Verification items for the finished model (mm, model axes). Face numbers are marked on the shaded views. A direction names the side the tool comes from. Coordinates: 2 decimals unless noted, no trailing zeros. Order: outer loops, then holes, each group sorted by start corner. A loop starts at its lowest first (then second) coordinate and runs counter-clockwise, first axis right, second up. Notation, with made-up numbers: (67.25, -1.5) -> (117.25, -1.5) arc R21 ccw to (117.25, 33.5) -> close; hole circle Ø10 at (-8.5, -32). An arc over 180 degrees is marked (long way). Write item = value, one per line. Start each with the question number.
from build123d import *

# Parameters (mm, degrees)
SKETCH1_W           = 8.89
SKETCH1_H           = 11.2776
SKETCH1_R           = 2.54
BOSS_EXTRUDE1_DEPTH = 2.54
SKETCH4_W           = 17.78
SKETCH4_H           = 11.43
SKETCH4_R           = 2.54
BOSS_EXTRUDE2_DEPTH = 2.54


with BuildPart() as part:
    # Sketch1 → Boss-Extrude1 (new body)
    with BuildSketch(Plane(origin=(0, 0, 0), x_dir=(1, 0, 0), z_dir=(0, 1, 0))):
        with Locations((-4.445, -5.6388)):
            Rectangle(SKETCH1_W, SKETCH1_H)
        with Locations((-4.445, -4.3688)):
            Circle(SKETCH1_R, mode=Mode.SUBTRACT)
    extrude(amount=BOSS_EXTRUDE1_DEPTH)

    # Sketch4 → Boss-Extrude2 (add)
    with BuildSketch(Plane.XY.offset(11.2776)):
        with Locations((-8.89, 5.715)):
            Rectangle(SKETCH4_W, SKETCH4_H)
        with Locations((-13.335, 6.985)):
            Circle(SKETCH4_R, mode=Mode.SUBTRACT)
    extrude(amount=-BOSS_EXTRUDE2_DEPTH)


solid = part.part
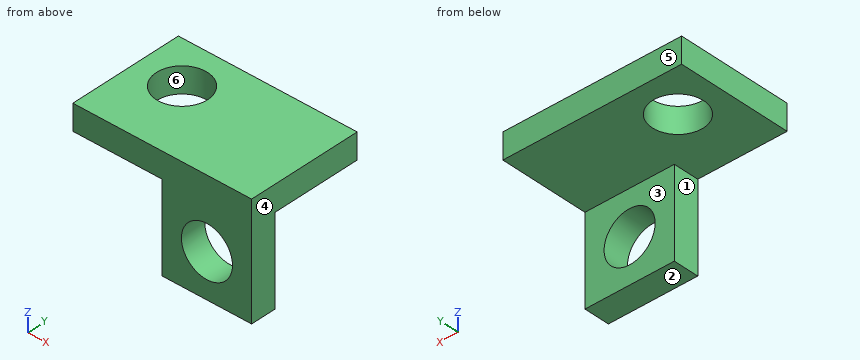
Item 1: Section check B-B (y = 7.25). Record the boundary of the cut face in (x, z).
Item 2: Section check A-A (x = -2.75). Record the boundary of the cut face in (y, z).
Item 3: Tool access check on the marked faces 1, 2 and 3. Record the directions out of +Z, -Z, +X, -X, +Y, -Y that give a thin tool (end or side, any length) a straight path to the whole face; none if there is none.
Item 4: Section check D-D (y = 1.5). Record the boundary of the cut face in (x, z) (3 decimals).
Item 5: Section check C-C (z = 5.25). Record the boundary of the cut face in (x, y).
Item 6: Thickness scan on line 1 (Y direction, x = -7.5, z = 1); line 2 (Z direction, x = -11, y = 2); line 3 (X direction, y = 1.75, z = 0.75). Record the ranges inside material, lowest first.
Item 7: Gauge pin test, flat ends, axial feed: P1, Ø4, axis at x = -4.44, z = 4.37, coming from the +Y side; P2, Ø2.5, axis at x = -4, z = 3, coming from the +Y side; P3, Ø0.8, axis at y = 2, z = 2.5, coming from the -X side; P4, Ø6.5, axis at x = -13.335, y = 6.985, coming from the +Z side. Record the tip position at first contact, or that the pin passes through.
Item 8: Mould release check, pull along Y, two halves, no side actions. Record for the marked faces 4, 5 and 6: pulls with the +Y half, pulls with the -Y half, needs draft (parallel to the pull), parting line crosses it, or undercut.
Filled sheet:
q1.outline = (-17.78, 8.74) -> (-15.86, 8.74) -> (-15.86, 11.28) -> (-17.78, 11.28) -> close; (-10.81, 8.74) -> (0, 8.74) -> (0, 11.28) -> (-10.81, 11.28) -> close
q2.outline = (0, 0) -> (2.54, 0) -> (2.54, 2.48) -> (0, 2.48) -> close; (0, 6.26) -> (2.54, 6.26) -> (2.54, 8.74) -> (11.43, 8.74) -> (11.43, 11.28) -> (0, 11.28) -> close
q3.face_1 = -Z, -X, +Y, -Y
q3.face_2 = -Z, +X, -X, +Y, -Y
q3.face_3 = -Z, +X, -X, +Y
q4.outline = (-17.78, 8.738) -> (-8.89, 8.738) -> (-8.89, 0) -> (0, 0) -> (0, 11.278) -> (-17.78, 11.278) -> close; hole circle Ø5.08 at (-4.445, 4.369)
q5.outline = (-8.89, 0) -> (-6.83, 0) -> (-6.83, 2.54) -> (-8.89, 2.54) -> close; (-2.06, 0) -> (0, 0) -> (0, 2.54) -> (-2.06, 2.54) -> close
q6.line_1 = 0 to 2.54
q6.line_2 = 8.74 to 11.28
q6.line_3 = -8.89 to 0
q7.P1 = through
q7.P2 = 2.54
q7.P3 = -8.89
q7.P4 = 11.28
q8.face_4 = needs draft
q8.face_5 = pulls with the +Y half
q8.face_6 = undercut
